Verification items for the finished model (mm, model axes). Give positions to 0.01 mm unless a question says otherwise; leave off trailing zeros. Loops run counter-clockwise (first coordinate to the right, second up) from the corner with the lowest first, then second, coordinate; pieces in that order, holes last. Notation, with made-up numbers: (-31, 82) - (-4, 82) arc R30 cw to (-4, 109) - close; hole circle Ø6 at (42, 55.5). An arc over 180 degrees is marked (long way). One line per question, with ' | ' between items. Start each with the question number.
1. Section check C-C, the plane x = 7. Enter the section's corners in (y, z) (3 decimals).
2. Section check D-D, the plane z = -14. Enter the section's corners in (x, y).
3. Depth check by flat-ended pin: pin 1 Ø2.5 at (x, z) = (-7.69, 6.92) entering from +Y. Enter the tip coordinate at first touch or a pass-through.
4. Section check A-A, the plane x = 0. Enter the section's corners in (y, z), then the cut area to 4 significant figures.
5. Thickness scan on line 1 along Z through (x, y) = (0, -0.25); line 2 along X through (y, z) = (-0.25, 9.5); line 3 along Z through (x, y) = (-0.5, -0.35). Record the ranges inside material, lowest first. Write a range as from..to.
6. Section check B-B, the plane z = 0. Enter the section's corners in (x, y).
7. Mould release check, pull along X, two halves, no side actions. Record for faces 1 (the face through (0, -0.5, -4)), 2 (the face through (-4.64, -0.25, 7.5)), 3 (the face through (-4.336, -0.246, -19.524)): +X half, -X half, draft (parallel to the pull), parting line (faces both ways), or undercut.
from build123d import *

# Parameters (mm, degrees)
F0_R           = 20
F1_DEPTH       = 0.5
F3_D           = 2.5
F4_R           = 2
F5_DEPTH       = 25.4
F7_D           = 0.5
F7_CSINK_D     = 1
F7_CSINK_ANGLE = 90
F9_D           = 2


with BuildPart() as f1:
    # F0 (on Front) → F1 (new body)
    with BuildSketch(Plane.XZ):
        Circle(F0_R)
    extrude(amount=F1_DEPTH)

    # F3 (through all)
    with Locations(Plane.XZ.offset(0.5)):
        with Locations((0, 0)):
            Hole(F3_D / 2)

    # F4 (on face) → F5 (cut)
    with BuildSketch(Plane.XZ.offset(0.5)):
        with Locations((-7.690389, 6.924457)):
            Circle(F4_R)
        with Locations((-4.209089, 9.453769)):
            Circle(F4_R)
        with Locations((0, 10.348439)):
            Circle(F4_R)
        with Locations((4.209089, 9.453769)):
            Circle(F4_R)
        with Locations((7.690389, 6.924457)):
            Circle(F4_R)
    extrude(amount=-F5_DEPTH, mode=Mode.SUBTRACT)

    # F7 (through all)
    with Locations(Plane.XZ.offset(0.5)):
        with Locations((13.66825, -12.708602)):
            CounterSinkHole(F7_D / 2, F7_CSINK_D / 2, counter_sink_angle=F7_CSINK_ANGLE)

    # F9 (through all)
    with Locations(Plane.XZ.offset(0.5)):
        with Locations((-11.675261, -5.019424)):
            Hole(F9_D / 2)


solid = f1.part
Results list:
1) outline: (-0.5, -18.735) - (0, -18.735) - (0, 5.047) - (-0.5, 5.047) - close; (-0.5, 8.802) - (0, 8.802) - (0, 18.735) - (-0.5, 18.735) - close
2) outline: (-14.28, -0.5) - (14.28, -0.5) - (14.28, 0) - (-14.28, 0) - close
3) pin 1: through
4) outline: (-0.5, -20) - (0, -20) - (0, -1.25) - (-0.5, -1.25) - close; (-0.5, 1.25) - (0, 1.25) - (0, 8.35) - (-0.5, 8.35) - close; (-0.5, 12.35) - (0, 12.35) - (0, 20) - (-0.5, 20) - close | area: 16.75 mm²
5) line 1: -20..-1.25, 1.25..8.35, 12.35..20 | line 2: -17.6..-6.21, -2.21..-1.81, 1.81..2.21, 6.21..17.6 | line 3: -19.99..-1.15, 1.15..8.41, 12.28..19.99
6) outline: (-20, -0.5) - (-1.25, -0.5) - (-1.25, 0) - (-20, 0) - close; (1.25, -0.5) - (20, -0.5) - (20, 0) - (1.25, 0) - close
7) face 1: draft | face 2: undercut | face 3: parting line
